Here's the drawing with two shaded views (mm, measured from the low corner). I have some questions. A direction names the side the tool comes from. Round coordinates to 2 decimals unless told otherwise and drop trailing zeros. Order: outer loops, then holes, each group sorted by start corner. A loop starts at its lowest first (then second) coordinate and runs counter-clockwise, first axis right, second up. Notation, with made-up numbers: (34, 53) - (60, 53) arc R29 ccw to (60, 81) - close; hole circle Ø9 at (4.5, -30.5). An arc over 180 degrees is marked (long way). One line per item, written item: value.
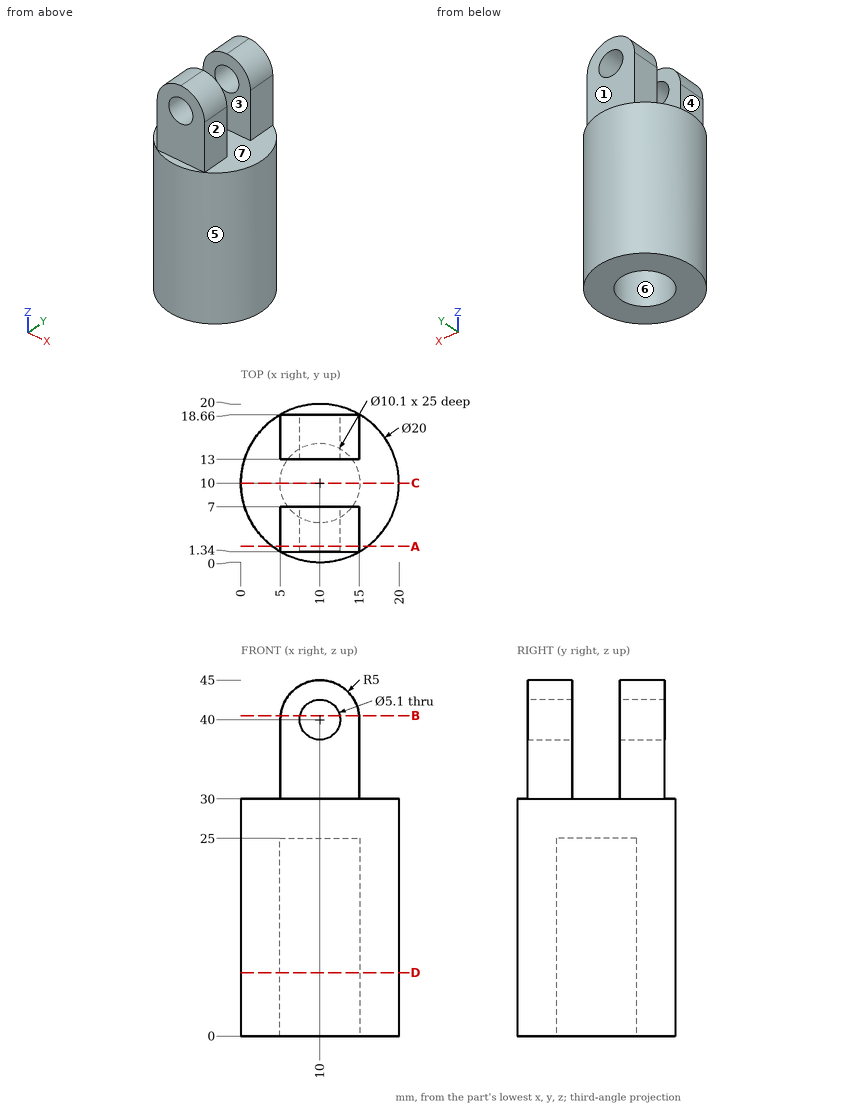
Q1. Which directions (+Z, -Z, +X, -X, +Y, -Y) give clear straight access to the entire face, cutting with the end or side of a thin tool? Please do the marked faces 1, 2, 3 and 4.
Results list:
face 1: +Z, +X, -X, +Y
face 2: +Z, +X, +Y, -Y
face 3: +Z, +X, -X
face 4: +Z, -X, +Y, -Y
Q2. We'd pull the mould along X, two halves only. Please class the marked faces 5, 6 and 7: released by +X, released by -X, zero draft, split by the parting line, or undercut.
Results list:
face 5: split by the parting line
face 6: undercut
face 7: zero draft
Q3. If we section it at B-B, the plane z = 40.5: Please give me the cut outline in (x, y) (1 decimal).
Results list:
outline: (5, 1.3) - (7.5, 1.3) - (7.5, 7) - (5, 7) - close; (5, 13) - (7.5, 13) - (7.5, 18.7) - (5, 18.7) - close; (12.5, 1.3) - (15, 1.3) - (15, 7) - (12.5, 7) - close; (12.5, 13) - (15, 13) - (15, 18.7) - (12.5, 18.7) - close
Q4. If we section it at A-A, the plane y = 2: Please give me the cut outline in (x, z).
Results list:
outline: (4, 0) - (16, 0) - (16, 30) - (15, 30) - (15, 40) arc R5 ccw to (5, 40) - (5, 30) - (4, 30) - close; hole circle Ø5.1 at (10, 40)
Q5. If we section it at D-D, the plane z = 8: Please give me the cut outline in (x, y), then the cut area to 3 significant figures.
Results list:
outline: circle Ø20 at (10, 10); hole circle Ø10.1 at (10, 10)
area: 234 mm²
Q6. If I drill on line 1 along X through (y, z) = (5.3, 40); line 2 along Y through (x, z) = (10, 9.25); line 3 along Y through (x, z) = (8.25, 34), over which ranges is the centre line in solid material (lowest first)?
Results list:
line 1: 5 to 7.45, 12.55 to 15
line 2: 0 to 4.95, 15.05 to 20
line 3: 1.34 to 7, 13 to 18.66
Q7. If we section it at C-C, the plane y = 10: Please give me the cut outline in (x, z).
Results list:
outline: (0, 0) - (4.95, 0) - (4.95, 25) - (15.05, 25) - (15.05, 0) - (20, 0) - (20, 30) - (0, 30) - close
Q8. Will these pins go through, and if not, where does the flat tip stop? pin 1 (6 mm diameter, centred on x = 17.5, z = 4.5, fed in from -Y); pin 2 (6 mm diameter, centred on x = 10, y = 10, fed in from -Z); pin 3 (11 mm diameter, centred on x = 11.5, z = 36.5, fed in from -Y); pin 4 (4.5 mm diameter, centred on x = 10, z = 40, fed in from -Y).
Results list:
pin 1: y = 1.07
pin 2: z = 25
pin 3: y = 1.34
pin 4: through
